from build123d import *

# Parameters (mm, degrees)
ESQUISSE1_W      = 8
ESQUISSE1_H      = 8
ESQUISSE1_R      = 1.5
EXTRUSION1_DEPTH = 1
ESQUISSE2_W      = 1
ESQUISSE2_H      = 8
EXTRUSION2_DEPTH = 7
EXTRUSION3_REACH = 10
ESQUISSE3_R      = 1.5


with BuildPart() as part:
    # Esquisse1 → Extrusion1 (new body)
    with BuildSketch(Plane(origin=(0, 0, 0), x_dir=(1, 0, 0), z_dir=(0, 1, 0))):
        with Locations((4, 4)):
            Rectangle(ESQUISSE1_W, ESQUISSE1_H)
        with Locations((4, 4)):
            Circle(ESQUISSE1_R, mode=Mode.SUBTRACT)
    extrude(amount=EXTRUSION1_DEPTH)

    # Esquisse2 → Extrusion2 (add)
    with BuildSketch(Plane(origin=(0, 1, 0), x_dir=(1, 0, 0), z_dir=(0, 1, 0))):
        with Locations((7.5, 4)):
            Rectangle(ESQUISSE2_W, ESQUISSE2_H)
    extrude(amount=EXTRUSION2_DEPTH)

    # Esquisse3 → Extrusion3 (cut, up to next)
    with BuildSketch(Plane(origin=(8, 0, 0), x_dir=(0, 0, -1), z_dir=(1, 0, 0)), mode=Mode.PRIVATE) as extrusion3_sk1:
        with Locations((4, 4)):
            Circle(ESQUISSE3_R)
    extrusion3_tool1 = extrude(extrusion3_sk1.sketch, amount=-EXTRUSION3_REACH, mode=Mode.PRIVATE) & part.part
    add(extrusion3_tool1.solids().sort_by_distance((8, 4, -4))[0], mode=Mode.SUBTRACT)


solid = part.part
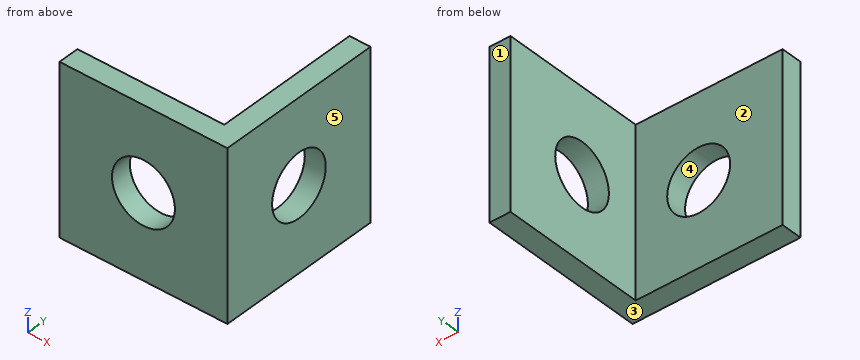
Build history of the part. All positions in model axes, mm. Face numbers are marked on the shaded views. A direction names the side the tool comes from. Round coordinates to 2 decimals unless told otherwise and drop trailing zeros. Loops run counter-clockwise (first coordinate to the right, second up) from the corner with the lowest first, then second, coordinate; pieces in that order, holes last. Notation, with made-up numbers: (16.5, 86) -> (69.5, 86) arc R15 cw to (69.5, 98) -> close; hole circle Ø3 at (35, 77.25). An arc over 180 degrees is marked (long way). Answer in a Markdown table with one row per item.
Item 1: Saw through at A-A (y = 4). Write the cut outline in (x, z), and give its area (3 significant figures).
Answers below:
| item | result |
|---|---|
| outline | (7, -8) -> (8, -8) -> (8, -5.5) -> (7, -5.5) -> close; (7, -2.5) -> (8, -2.5) -> (8, 0) -> (7, 0) -> close |
| area | 5.00 mm² |
Item 2: Saw through at D-D (z = -3). Write the cut outline in (x, y).
Answers below:
| item | result |
|---|---|
| outline | (0, 0) -> (2.88, 0) -> (2.88, 1) -> (0, 1) -> close; (5.12, 0) -> (8, 0) -> (8, 2.88) -> (7, 2.88) -> (7, 1) -> (5.12, 1) -> close; (7, 5.12) -> (8, 5.12) -> (8, 8) -> (7, 8) -> close |
Item 3: Saw through at C-C (x = 4). Write the cut outline in (y, z), and give its area (3 significant figures).
Answers below:
| item | result |
|---|---|
| outline | (0, -8) -> (1, -8) -> (1, -5.5) -> (0, -5.5) -> close; (0, -2.5) -> (1, -2.5) -> (1, 0) -> (0, 0) -> close |
| area | 5.00 mm² |
Item 4: Which spindle directions (+Z, -Z, +X, -X, +Y, -Y) get a long thin tool onto all of the face, cutting with end or side? Do the marked faces 1 and 2. Say none if no direction does.
Answers below:
| item | result |
|---|---|
| face 1 | +Z, -Z, +X, -X, +Y |
| face 2 | +Z, -Z, -X, +Y |
Item 5: Mould opens along Z. For the marked faces 3, 4 and 5 say: +Z half, -Z half, draft (parallel to the pull), parting line (faces both ways), or undercut.
Answers below:
| item | result |
|---|---|
| face 3 | -Z half |
| face 4 | undercut |
| face 5 | draft |
Item 6: Saw through at B-B (z = -4). Write the cut outline in (x, y), and give its area (3 significant figures).
Answers below:
| item | result |
|---|---|
| outline | (0, 0) -> (2.5, 0) -> (2.5, 1) -> (0, 1) -> close; (5.5, 0) -> (8, 0) -> (8, 2.5) -> (7, 2.5) -> (7, 1) -> (5.5, 1) -> close; (7, 5.5) -> (8, 5.5) -> (8, 8) -> (7, 8) -> close |
| area | 9.00 mm² |
Item 7: Pin check, flat tips, straight feed: pin 1 (1 mm diameter, centred on y = 6, z = -4, fed in from -X); pin 2 (2 mm diameter, centred on x = 3.5, z = -5, fed in from +Y). Stop position of each tip, or through.
Answers below:
| item | result |
|---|---|
| pin 1 | stops at x = 7 |
| pin 2 | stops at y = 1 |
Item 8: Drill centre lines: L1, parallel to Z at x = 4, y = 0.6; L2, parallel to Y at x = 7.7, z = -4. Where is each one in solid material? Low to high. Write a range as [from, to].
Answers below:
| item | result |
|---|---|
| L1 | z = [-8, -5.5], [-2.5, 0] |
| L2 | y = [0, 2.5], [5.5, 8] |
